CAD build for the part. Positions are in the model's coordinates, mm. Coordinates: 2 decimals unless noted, no trailing zeros. Order: outer loops, then holes, each group sorted by start corner. A loop starts at its lowest first (then second) coordinate and runs counter-clockwise, first axis right, second up. Notation, with made-up numbers: (44, -20.75) - (84, -20.75) arc R15 cw to (84, 6.25) - close; hole circle Ø6 at (65.25, 51). An arc over 180 degrees is marked (long way). Return JSON: item names as keys, results as strings.
Autodesk Inventor part; units mm, degrees
ref_plane "YZ Plane" through (0, 0, 0) normal (1, 0, 0) x (0, 1, 0)
ref_plane "XZ Plane" through (0, 0, 0) normal (0, 1, 0) x (-1, 0, 0)
ref_plane "XY Plane" through (0, 0, 0) normal (0, 0, 1) x (1, 0, 0)
sketch "Sketch2" plane through (0, 0, 0) normal (0, 0, 1) x (1, 0, 0)
  circle A0 centre (-2.0274, 2.6474) radius 6.8
  ellipse E0 centre (-2.0274, 2.6474) end of major axis (-2.0274, -4.5526) minor radius 11.9605
  circle A1 centre (-2.0274, 2.6474) radius 5.8
  point P0 (0, 0)
  dimension "d25" = 1
extrude "Extrusion5" add sketch "Sketch2" against normal blind 80.6 contours A0 | A1
extrude "Extrusion6" add sketch "Sketch2" against normal blind 1 contours E0
extrude "Extrusion7" cut sketch "Sketch2" against normal blind 79.6 contours A1
properties part number "seringa outer" material "Glass"
Item 1: Band-saw the part on A-A, the plane z = -66. List the corners of the cut face in (x, y), then the cut area to 3 significant figures.
Findings below:
{"outline": "circle Ø13.6 at (-2.03, 2.65); hole circle Ø11.6 at (-2.03, 2.65)", "area": "39.6 mm²"}
Item 2: Mould opens along X. For faces 1 (the flat face through (3.1, -2.1, -1)), 2 (the cylindrical face through (-6.3, 6.57, -39.24)), 3 (the cylindrical face through (-7.424, -1.49, -40.243)), 4 (the flat face through (-2, 3, -79.6)) say: released by +X, released by -X, zero draft, split by the parting line, or undercut.
Findings below:
{"face 1": "zero draft", "face 2": "undercut", "face 3": "split by the parting line", "face 4": "undercut"}
Item 3: Wall check: L1, parallel to Z at x = 7.75, y = 5; L2, parallel to Z at x = -2, y = 6.5; L3, parallel to X at y = 8, z = -21.5. Give the ranges that are in metal, low to high. Write a range as [from, to].
Findings below:
{"L1": "z = [-1, 0]", "L2": "z = [-80.6, -79.6]", "L3": "x = [-6.22, -4.26], [0.21, 2.17]"}
Item 4: Drop flat-ended pins along their axis: P1, Ø8, axis at y = 1, z = -8.5, coming from the +X side; P2, Ø5, axis at x = 6, y = 5.5, coming from the -Z side; P3, Ø8, axis at y = 1, z = -61, coming from the -X side; P4, Ø8, axis at y = 8, z = -14, coming from the +X side. Give the stop position or say it passes through.
Findings below:
{"P1": "stops at x = 4.77", "P2": "stops at z = -80.6", "P3": "stops at x = -8.83", "P4": "stops at x = 4.64"}
